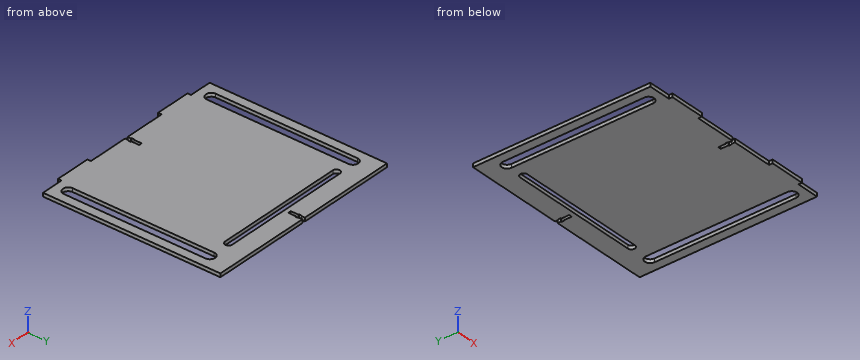
```python
from build123d import *

# Parameters (mm, degrees)
BOSS_EXTRU_1_DEPTH      = 5
ENL_V_MAT_EXTRU_1_DEPTH = 328.095566225


with BuildPart() as part:
    # Esquisse1 → Boss.-Extru.1 (new body)
    with BuildSketch(Plane.XY):
        Polygon((-51.387751479, -19.023668639), (-19.917751479, -19.023668639), (-19.917751479, -24.023668639), (30.082248521, -24.023668639), (30.082248521, -19.023668639), (87.982248521, -19.023668639), (87.982248521, -14.023668639), (86.982248521, -14.023668639), (86.982248521, -10.023668639), (87.982248521, -10.023668639), (87.982248521, 0.976331361), (92.182248521, 0.976331361), (92.182248521, -10.023668639), (93.182248521, -10.023668639), (93.182248521, -14.023668639), (92.182248521, -14.023668639), (92.182248521, -19.023668639), (150.082248521, -19.023668639), (150.082248521, -24.023668639), (200.082248521, -24.023668639), (200.082248521, -19.023668639), (231.552248521, -19.023668639), (231.552248521, 230.976331361), (200.082248521, 230.976331361), (150.082248521, 230.976331361), (92.182248521, 230.976331361), (92.182248521, 225.976331361), (93.182248521, 225.976331361), (93.182248521, 221.976331361), (92.182248521, 221.976331361), (92.182248521, 210.976331361), (87.982248521, 210.976331361), (87.982248521, 221.976331361), (86.982248521, 221.976331361), (86.982248521, 225.976331361), (87.982248521, 225.976331361), (87.982248521, 230.976331361), (30.082248521, 230.976331361), (-19.917751479, 230.976331361), (-51.387751479, 230.976331361), align=None)
    extrude(amount=BOSS_EXTRU_1_DEPTH)

    # Esquisse2 → Enlèv. mat.-Extru.1 (cut, through all)
    with BuildSketch(Plane(origin=(0, 0, 0), x_dir=(-1, 0, 0), z_dir=(0, 0, -1))):
        with BuildLine():
            Line((-204.052248521, 199.47878379), (-204.052248521, 0))
            ThreePointArc((-204.052248521, 0), (-211.552248521, -7.5), (-219.052248521, 0))
            Line((-219.052248521, 0), (-219.052248521, 199.47878379))
            ThreePointArc((-219.052248521, 199.47878379), (-211.552248521, 206.97878379), (-204.052248521, 199.47878379))
        make_face()
        with BuildLine():
            Line((-179.579242919, 204.47878379), (3.336091455, 204.47878379))
            ThreePointArc((3.336091455, 204.47878379), (8.336091455, 199.47878379), (3.336091455, 194.47878379))
            Line((3.336091455, 194.47878379), (-179.579242919, 194.47878379))
            ThreePointArc((-179.579242919, 194.47878379), (-184.579242919, 199.47878379), (-179.579242919, 204.47878379))
        make_face()
        with BuildLine():
            Line((38.887751479, 199.47878379), (38.887751479, 0))
            ThreePointArc((38.887751479, 0), (31.387751479, -7.5), (23.887751479, 0))
            Line((23.887751479, 0), (23.887751479, 199.47878379))
            ThreePointArc((23.887751479, 199.47878379), (31.387751479, 206.97878379), (38.887751479, 199.47878379))
        make_face()
    extrude(amount=-ENL_V_MAT_EXTRU_1_DEPTH, mode=Mode.SUBTRACT)


solid = part.part
```
Work out the finished part from the listing and answer in its coordinate system (mm). Coordinates: 2 decimals unless noted, no trailing zeros. Order: outer loops, then holes, each group sorted by start corner. A loop starts at its lowest first (then second) coordinate and runs counter-clockwise, first axis right, second up. Notation, with made-up numbers: M -16,46.5 L 27,46.5 A33 cw 27,74.5 Z; hole C 72,-30 d8. An arc over 180 degrees is marked long. Use CSV: the item, a comma, the result in double quotes.
1) Consider line 1 (Y direction, x = 93, z = 4.3); line 2 (X direction, y = 159, z = 3.85); line 3 (X direction, y = 200, z = 2.2). Determine where each line is inside the solid, lowest interval first. Write a range as [from, to].
Worked out:
line 1,"y = [-19.02, -14.02], [-10.02, 194.48], [204.48, 221.98], [225.98, 230.98]"
line 2,"x = [-51.39, -38.89], [-23.89, 204.05], [219.05, 231.55]"
line 3,"x = [-51.39, -38.87], [-23.91, -8.31], [184.55, 204.07], [219.03, 231.55]"
2) Flat-ended cylindrical pins translate along their axes: pin 1 Ø0.5 at (x, z) = (87.5, 3.5) entering from -Y; pin 2 Ø2.5 at (y, z) = (-22.5, 3.5) entering from +X. Find the tip coordinate at first contact, or state that the pin passes through.
Worked out:
pin 1,"stops at y = -19.02"
pin 2,"stops at x = 200.08"
3) Section C-C on z = 2.3 is taken. Count the separate pieces of the cut face and the enclosed holes in it, plus the area to 3 significant figures.
Worked out:
separate pieces,"1"
enclosed holes,"3"
area,"62,800 mm^2"
4) Section A-A on y = 159 is taken. Write down the section's boundary in (x, z), plus the area to 3 significant figures.
Worked out:
outline,"M -51.39,0 L -38.89,0 L -38.89,5 L -51.39,5 Z; M -23.89,0 L 204.05,0 L 204.05,5 L -23.89,5 Z; M 219.05,0 L 231.55,0 L 231.55,5 L 219.05,5 Z"
area,"1,260 mm^2"
5) Section B-B on x = 53 is taken. Write down the section's boundary in (y, z), plus the area to 3 significant figures.
Worked out:
outline,"M -19.02,0 L 194.48,0 L 194.48,5 L -19.02,5 Z; M 204.48,0 L 230.98,0 L 230.98,5 L 204.48,5 Z"
area,"1,200 mm^2"
